Verification items for the finished model (mm, model axes). A direction names the side the tool comes from. Give positions to 0.01 mm unless a question says otherwise; leave off trailing zeros. Write each loop counter-clockwise with the first axis right and the second up, starting at its lowest first coordinate (ties: lowest second). Pieces come first, ordered by that corner, then holes. Notation, with made-up numbers: (-18.5, -38.5) -> (17.5, -38.5) arc R11 cw to (17.5, -28.5) -> close; hole circle Ø4 at (-27.75, 69.25). An arc over 180 degrees is marked (long way). Write item = value, one per line.
from build123d import *

# Parameters (mm, degrees)
SKETCH1_W                            = 30
SKETCH1_H                            = 20
BOSS_EXTRUDE1_DEPTH                  = 10
SKETCH3_R                            = 2
CUT_EXTRUDE1_DEPTH                   = 27.925824036
SKETCH4_R                            = 2
CUT_EXTRUDE2_DEPTH                   = 27.925824036
FILLET1_R                            = 4
SKETCH5_R                            = 3.9
BOSS_EXTRUDE2_DEPTH                  = 9.5
BOSS_EXTRUDE2_DIRECTION_2_REACH      = 22.616
BOSS_EXTRUDE2_DIRECTION_2_END_RADIUS = 4
CUT_EXTRUDE3_DEPTH                   = 21.615528249
FILLET3_R                            = 3
BOSS_EXTRUDE3_START                  = -0.291901
BOSS_EXTRUDE3_DEPTH                  = 3.291901
SKETCH8_R                            = 2.25
CUT_EXTRUDE4_DEPTH                   = 8
CUT_EXTRUDE5_DEPTH                   = 32.705677897
CUT_EXTRUDE6_DEPTH                   = 32.705677897


with BuildPart() as part:
    # Sketch1 → Boss-Extrude1 (new body)
    with BuildSketch(Plane.XY):
        Rectangle(SKETCH1_W, SKETCH1_H)
    extrude(amount=BOSS_EXTRUDE1_DEPTH)

    # Sketch3 → Cut-Extrude1 (cut, through all)
    with BuildSketch(Plane(origin=(0, 10, 0), x_dir=(1, 0, 0), z_dir=(0, 1, 0))):
        with Locations(Location((11, -5, 0), (0, 0, 270))):
            Circle(SKETCH3_R)
    extrude(amount=-CUT_EXTRUDE1_DEPTH, mode=Mode.SUBTRACT)

    # Sketch4 → Cut-Extrude2 (cut, through all)
    with BuildSketch(Plane.XZ.offset(10)):
        with Locations(Location((-9, 5, 0), (0, 0, 270))):
            Circle(SKETCH4_R)
    extrude(amount=-CUT_EXTRUDE2_DEPTH, mode=Mode.SUBTRACT)

    # Fillet1
    fillet1_edges = [part.edges().sort_by_distance(p)[0] for p in [
        (15, 0, 10),
        (15, 0, 0),
    ]]
    fillet(fillet1_edges, radius=FILLET1_R)

    # Sketch5 → Boss-Extrude2 (add)
    with BuildSketch(Plane.XY.offset(10)):
        with Locations(Location((11, 0, 0), (0, 0, 180))):
            Circle(SKETCH5_R)
    extrude(amount=BOSS_EXTRUDE2_DEPTH)

    # Boss-Extrude2 direction 2: up to this cylinder (the profile starts outside it)
    boss_extrude2_direction_2_end = Plane(origin=(11, 0, 6), z_dir=(0, -1, 0)) * Cylinder(BOSS_EXTRUDE2_DIRECTION_2_END_RADIUS, 54.232, mode=Mode.PRIVATE)
    # Sketch5 → Boss-Extrude2 direction 2 (add, up to the surface)
    with BuildSketch(Plane.XY.offset(10), mode=Mode.PRIVATE) as boss_extrude2_direction_2_sk1:
        with Locations(Location((11, 0, 0), (0, 0, 180))):
            Circle(SKETCH5_R)
    boss_extrude2_direction_2_tool1 = extrude(boss_extrude2_direction_2_sk1.sketch, amount=-BOSS_EXTRUDE2_DIRECTION_2_REACH, mode=Mode.PRIVATE) - boss_extrude2_direction_2_end
    add(boss_extrude2_direction_2_tool1.solids().sort_by_distance((11, 0, 10))[0])
    add(boss_extrude2_direction_2_tool1.solids().sort_by_distance((11, 0, 10))[1])

    # Sketch6 → Cut-Extrude3 (cut, through all)
    with BuildSketch(Plane.XY.offset(10)):
        Polygon((-15, -6), (-2.46092253, -6), (5, 10), (-15, 10), align=None)
    extrude(amount=-CUT_EXTRUDE3_DEPTH, mode=Mode.SUBTRACT)

    # Fillet3
    fillet3_edges = [part.edges().sort_by_distance(p)[0] for p in [
        (1.269538735, 2, 0),
        (1.269538735, 2, 10),
    ]]
    fillet(fillet3_edges, radius=FILLET3_R)

    # Sketch7 → Boss-Extrude3 (add)
    with BuildSketch(Plane.XY.offset(10).offset(BOSS_EXTRUDE3_START)):
        with BuildLine():
            Line((12.5, 5.499090834), (12.5, -5.499090834))
            ThreePointArc((12.5, -5.499090834), (5.3, 0), (12.5, 5.499090834))
        make_face()
    extrude(amount=BOSS_EXTRUDE3_DEPTH)

    # Sketch8 → Cut-Extrude4 (cut)
    with BuildSketch(Plane.XY.offset(19.5)):
        with Locations((11, 0)):
            Circle(SKETCH8_R)
    extrude(amount=-CUT_EXTRUDE4_DEPTH, mode=Mode.SUBTRACT)

    # Sketch9 → Cut-Extrude5 (cut, through all)
    with BuildSketch(Plane.XZ.offset(10)):
        with BuildLine():
            Line((-9, 10), (-15, 10))
            Line((-15, 10), (-15, 0))
            Line((-15, 0), (-9, 0))
            ThreePointArc((-9, 0), (-14, 5), (-9, 10))
        make_face()
    extrude(amount=-CUT_EXTRUDE5_DEPTH, mode=Mode.SUBTRACT)

    # Sketch10 → Cut-Extrude6 (cut, through all)
    with BuildSketch(Plane(origin=(0, 10, 0), x_dir=(1, 0, 0), z_dir=(0, 1, 0))):
        with BuildLine():
            Line((8.5, -4.5), (9.063508327, -4.5))
            ThreePointArc((9.063508327, -4.5), (9.015940607, -4.747991415), (9, -5))
            ThreePointArc((9, -5), (9.015940607, -5.252008585), (9.063508327, -5.5))
            Line((9.063508327, -5.5), (8.5, -5.5))
            Line((8.5, -5.5), (8.5, -4.5))
        make_face()
        with BuildLine():
            Line((10.5, -2.5), (10.5, -3.063508327))
            ThreePointArc((10.5, -3.063508327), (10.747991415, -3.015940607), (11, -3))
            ThreePointArc((11, -3), (11.252008585, -3.015940607), (11.5, -3.063508327))
            Line((11.5, -3.063508327), (11.5, -2.5))
            Line((11.5, -2.5), (10.5, -2.5))
        make_face()
        with BuildLine():
            Line((13.5, -4.5), (12.936491673, -4.5))
            ThreePointArc((12.936491673, -4.5), (12.984059393, -4.747991415), (13, -5))
            ThreePointArc((13, -5), (12.984059393, -5.252008585), (12.936491673, -5.5))
            Line((12.936491673, -5.5), (13.5, -5.5))
            Line((13.5, -5.5), (13.5, -4.5))
        make_face()
        with BuildLine():
            Line((11.5, -7.5), (11.5, -6.936491673))
            ThreePointArc((11.5, -6.936491673), (11.252008585, -6.984059393), (11, -7))
            ThreePointArc((11, -7), (10.747991415, -6.984059393), (10.5, -6.936491673))
            Line((10.5, -6.936491673), (10.5, -7.5))
            Line((10.5, -7.5), (11.5, -7.5))
        make_face()
    extrude(amount=-CUT_EXTRUDE6_DEPTH, mode=Mode.SUBTRACT)


solid = part.part
Item 1: Set-up check for faces 5 (the flat face through (12.5, -5, 11)), 6 (the flat face through (11, 0, 11.5)), 7 (the flat face through (3, -4, 10)), 8 (the flat face through (0, -10, 5)), 9 (the cylindrical face through (9.575, 0.14, 6.404)): record each of +Z, -Z, +X, -X, +Y, -Y from which the full face is reachable in a straight line by a thin tool's end or side.
Response values:
face_5 = +Z, +X, -Y
face_6 = +Z
face_7 = +Z, -X
face_8 = +Z, -Z, +X, -X, -Y
face_9 = +Y, -Y
Item 2: Sectioned sample at C-C on z = 14.5. Record the cut outline in (x, y).
Response values:
outline = circle Ø7.8 at (11, 0); hole circle Ø4.5 at (11, 0)
Item 3: Go/stop test with flat-tipped pins: P1, Ø0.5, axis at y = 0, z = 2.5, coming from the +X side; P2, Ø3, axis at x = -7, z = 4.5, coming from the +Y side; P3, Ø4, axis at x = 7, z = 16, coming from the -Y side; P4, Ø12, axis at x = -6.5, y = 0.5, coming from the -Z side. Record where each tip stops, or that it passes through.
Response values:
P1 = 14.8
P2 = -6
P3 = -3.35
P4 = through
Item 4: Sectioned sample at D-D on z = 9. Record the cut outline in (x, y).
Response values:
outline = (-12, -10) -> (13.65, -10) -> (13.65, -2.87) arc R3.9 ccw to (13.65, 2.87) -> (13.65, 10) -> (5.84, 10) -> (-1.62, -6) -> (-12, -6) -> close
Item 5: Sectioned sample at B-B on y = -8.5. Record the cut outline in (x, z).
Response values:
outline = (-9, 0) -> (11, 0) arc R4 ccw to (15, 4) -> (15, 6) arc R4 ccw to (11, 10) -> (-9, 10) arc R5 ccw to start; hole circle Ø4 at (-9, 5); hole (8.5, 4.5) -> (9.06, 4.5) arc R2 ccw to (10.5, 3.06) -> (10.5, 2.5) -> (11.5, 2.5) -> (11.5, 3.06) arc R2 ccw to (12.94, 4.5) -> (13.5, 4.5) -> (13.5, 5.5) -> (12.94, 5.5) arc R2 ccw to (11.5, 6.94) -> (11.5, 7.5) -> (10.5, 7.5) -> (10.5, 6.94) arc R2 ccw to (9.06, 5.5) -> (8.5, 5.5) -> close
Item 6: Material ranges on line 1 (X direction, y = -7.75, z = 5); line 2 (Y direction, x = 11, z = 16); line 3 (Z direction, x = 7.5, y = -6), recorded low to high.
Response values:
line_1 = -14 to -11, -7 to 8.5, 13.5 to 15
line_2 = -3.9 to -2.25, 2.25 to 3.9
line_3 = 0 to 10
Item 7: Mould release check, pull along Z, two halves, no side actions. Record for faces 1 (the cylindrical face through (14.98, 0.14, 6.39)), 2 (the flat face through (11, 0, 2.5)), 3 (the flat face through (11, 0, 7.5)), 4 (the flat face through (-6.7, -6, 5.1)): +Z half, -Z half, draft (parallel to the pull), parting line (faces both ways), or undercut.
Response values:
face_1 = +Z half
face_2 = undercut
face_3 = undercut
face_4 = draft
Item 8: Sectioned sample at A-A on z = 5. Record the cut outline in (x, y), then the cut area to 3 significant figures.
Response values:
outline = (-14, -10) -> (-11, -10) -> (-11, -6) -> (-14, -6) -> close; (-7, -10) -> (8.5, -10) -> (8.5, 10) -> (5, 10) -> (-2.46, -6) -> (-7, -6) -> close; (13.5, -10) -> (15, -10) -> (15, 10) -> (13.5, 10) -> close
area = 220 mm^2
